Input: part model. Units: mm. Frame: model coordinates. Face numbers are marked on the shaded views. A direction names the side the tool comes from. Coordinates: 2 decimals unless noted, no trailing zeros. Loops run counter-clockwise (first coordinate to the right, second up) from the corner with the lowest first, then second, coordinate; pieces in that order, holes last.
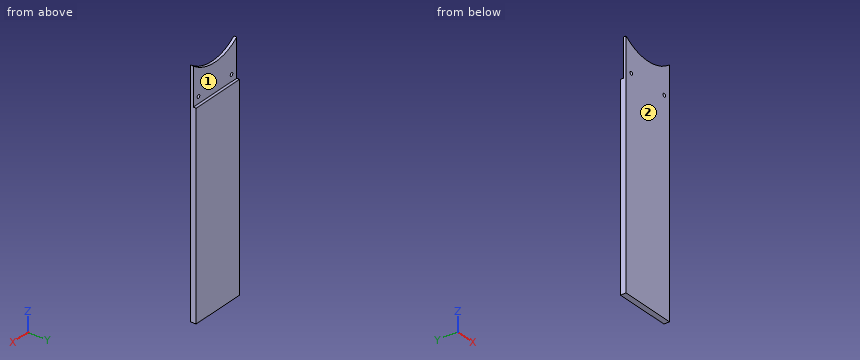
Autodesk Inventor part; units mm, degrees
ref_plane "YZ Plane" through (0, 0, 0) normal (1, 0, 0) x (0, 1, 0)
ref_plane "XZ Plane" through (0, 0, 0) normal (0, 1, 0) x (-1, 0, 0)
ref_plane "XY Plane" through (0, 0, 0) normal (0, 0, 1) x (1, 0, 0)
sketch "Esboço1" plane through (0, 0, 0) normal (0, 1, 0) x (-1, 0, 0)
  line L0 (-1.3226, 64.6966) -> (-1.3226, 176.6966) construction
  line L1 (-1.3226, 64.6966) -> (-1.3226, 179.6966) construction
  line L2 (23.6774, 24.6966) -> (-26.3226, 24.6966)
  line L3 (-26.3226, 24.6966) -> (-26.3226, -57.3034)
  line L4 (-26.3226, -57.3034) -> (23.6774, -57.3034)
  line L5 (23.6774, -57.3034) -> (23.6774, 24.6966)
  line L6 (23.6774, -57.3034) -> (-26.3226, -57.3034)
  line L7 (-26.3226, -57.3034) -> (-26.3226, -177.3034)
  line L8 (-26.3226, -177.3034) -> (23.6774, -177.3034)
  line L9 (23.6774, -177.3034) -> (23.6774, -57.3034)
  line L10 (23.6774, 24.6966) -> (23.6774, 33.4716)
  line L11 (-26.3226, 24.6966) -> (-26.3226, 33.4716)
  line L12 (23.6774, 24.6966) -> (-26.3226, 24.6966)
  line L13 (-26.3226, 24.6966) -> (-26.3226, -0.3034)
  line L14 (-26.3226, -0.3034) -> (23.6774, -0.3034)
  line L15 (23.6774, -0.3034) -> (23.6774, 24.6966)
  circle A0 centre (17.6774, 5.6966) radius 1.5
  circle A1 centre (17.6774, 5.6966) radius 2.75
  circle A2 centre (-20.3226, 5.6966) radius 1.5
  circle A3 centre (-20.3226, 5.6966) radius 2.75
  arc A4 (-26.3226, 33.4716) -> (23.6774, 33.4716) centre (-1.3226, 64.6966) ccw
  point P0 (0, 0)
  point P1 (-26.3226, -57.3034)
  dimension "d8" = 120
  dimension "d9" = 50
  dimension "d10" = 25
  dimension "d11" = 25
  dimension "d12" = 50
  dimension "d13" = 3
  dimension "d14" = 6
  dimension "d15" = 6
  dimension "d16" = 5.5
extrude "Extrusão1" add sketch "Esboço1" along normal blind 2.5 contours L5 L14 L3 L2 | L2 A4 L10 | L2 L11 A4 | A1 | A3
extrude "Extrusão2" add sketch "Esboço1" along normal blind 5 contours L5 L4 L3 L14 | L9 L8 L7 L4
properties part number "peca2_suporte"
Item 1: Section query D-D (x = -13). Output: boundary loops of the cut face in (y, z), then the cut area to 3 significant figures.
Result:
outline: (0, -177.3) - (5, -177.3) - (5, -0.3) - (2.5, -0.3) - (2.5, 27.35) - (0, 27.35) - close
area: 954 mm2
Item 2: Section query A-A (y = 3.7). Output: boundary loops of the cut face in (x, z).
Result:
outline: (-23.68, -177.3) - (26.32, -177.3) - (26.32, -0.3) - (-23.68, -0.3) - close
Item 3: Section query B-B (x = 5). Output: boundary loops of the cut face in (y, z), then the cut area to 3 significant figures.
Result:
outline: (0, -177.3) - (5, -177.3) - (5, -0.3) - (2.5, -0.3) - (2.5, 24.87) - (0, 24.87) - close
area: 948 mm2
Item 4: Line query: L1, parallel to Z at x = -17.5, y = 4.7; L2, parallel to Z at x = 1, y = 0.7; L3, parallel to Y at x = 7.5, z = 3. Output: solid intervals per line, ascending.
Result:
L1: z = -177.3 to -0.3
L2: z = -177.3 to 24.7
L3: y = 0 to 2.5
Item 5: Section query C-C (z = 20.5). Output: boundary loops of the cut face in (x, y), then the cut area to 3 significant figures.
Result:
outline: (-23.68, 0) - (26.32, 0) - (26.32, 2.5) - (-23.68, 2.5) - close
area: 125 mm2
Item 6: Reachability of the marked faces 1 and 2 from +Z, -Z, +X, -X, +Y, -Y: full face, straight path, thin tool, end or side. Return the list, or none.
Result:
face 1: +Z, +X, -X, +Y
face 2: +Z, -Z, +X, -X, -Y
Item 7: Contact query for flat-ended pins moving along their axis: P1, Ø10, axis at x = -8, z = 12, coming from the +Y side; P2, Ø10, axis at x = -2, z = -2, coming from the -Y side; P3, Ø2.5, axis at x = 20.32, z = 5.7, coming from the +Y side; P4, Ø1.2, axis at x = 0.5, y = 3, coming from the +Z side. Output: stop coordinate, or through.
Result:
P1: stops at y = 2.5
P2: stops at y = 0
P3: passes through
P4: stops at z = 24.71
